Work out the finished part from the listing and answer in its coordinate system (mm). Face numbers are marked on the shaded views. A direction names the side the tool comes from. Coordinates: 2 decimals unless noted, no trailing zeros. Loops run counter-clockwise (first coordinate to the right, second up) from the corner with the lowest first, then second, coordinate; pieces in that order, holes last.
```python
from build123d import *

# Parameters (mm, degrees)
SKETCH_W        = 110
SKETCH_H        = 80
PAD_DEPTH       = 50
SKETCH001_R     = 1
POCKET_DEPTH    = 48
FILLET_R        = 2
FILLET001_R     = 2
SKETCH002_R     = 2.55
SKETCH002_W     = 11.5
SKETCH002_H     = 19.1
POCKET001_DEPTH = 5
SKETCH003_R     = 2.55
POCKET002_DEPTH = 5
BOX_W           = 15
BOX_H           = 15
BOX_DEPTH       = 15


with BuildPart() as body:
    # Sketch → Pad (new body)
    with BuildSketch(Plane.XY):
        with Locations((55, 40)):
            Rectangle(SKETCH_W, SKETCH_H)
    extrude(amount=PAD_DEPTH)

    # Sketch001 (on Face6 of Pad) → Pocket (cut)
    with BuildSketch(Plane.XY.offset(50)):
        with Locations((6, 74)):
            Circle(SKETCH001_R)
        with Locations((104, 74)):
            Circle(SKETCH001_R)
        with Locations((104, 6)):
            Circle(SKETCH001_R)
        with Locations((6, 6)):
            Circle(SKETCH001_R)
        Polygon((2, 10), (10, 10), (10, 2), (100, 2), (100, 10), (108, 10), (108, 70), (100, 70), (100, 78), (10, 78), (10, 70), (2, 70), align=None)
    extrude(amount=-POCKET_DEPTH, mode=Mode.SUBTRACT)

    # Fillet
    fillet_edges = [body.edges().sort_by_distance(p)[0] for p in [
        (0, 80, 25),
        (0, 40, 0),
        (0, 0, 25),
        (55, 0, 0),
        (110, 0, 25),
        (110, 80, 25),
        (110, 40, 0),
        (55, 80, 0),
    ]]
    fillet(fillet_edges, radius=FILLET_R)

    # Fillet001
    fillet001_edges = [body.edges().sort_by_distance(p)[0] for p in [
        (100, 10, 26),
        (100, 70, 26),
        (10, 70, 26),
        (10, 10, 26),
    ]]
    fillet(fillet001_edges, radius=FILLET001_R)

    # Sketch002 (on Face22 of Fillet001) → Pocket001 (cut)
    with BuildSketch(Plane.YZ.offset(110)):
        with Locations((15, 27.5)):
            Circle(SKETCH002_R)
        with Locations((28.75, 27.5)):
            Rectangle(SKETCH002_W, SKETCH002_H)
    extrude(amount=-POCKET001_DEPTH, mode=Mode.SUBTRACT)

    # Sketch003 (on Face18 of Pocket001) → Pocket002 (cut)
    with BuildSketch(Plane.XZ):
        with Locations((95, 27.5)):
            Circle(SKETCH003_R)
    extrude(amount=-POCKET002_DEPTH, mode=Mode.SUBTRACT)


with BuildPart() as common:
    # Box → Box (new body)
    with BuildSketch(Plane(origin=(95, 0, 35), x_dir=(1, 0, 0), z_dir=(0, 0, 1))):
        with Locations((7.5, 7.5)):
            Rectangle(BOX_W, BOX_H)
    extrude(amount=BOX_DEPTH)

    # Common: intersect Body
    add(body.part, mode=Mode.INTERSECT)


solid = common.part
```
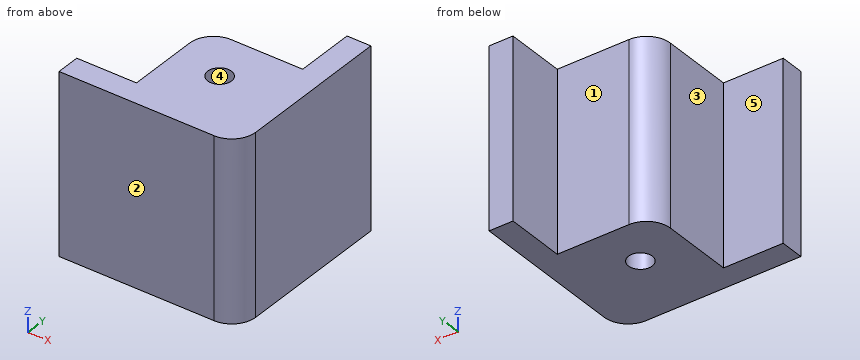
1. A cutting plane is placed at A-A, the plane y = 6. Give the vertices of the cut face in (x, z), then the cut area to 3 significant figures.
2. A cutting plane is placed at B-B, the plane x = 104. Give the vertices of the cut face in (y, z).
3. Determine the mould class of the marked faces 3, 4 and 5 for opening direction X: released by +X, released by -X, zero draft, split by the parting line, or undercut.
4. A cutting plane is placed at C-C, the plane z = 43. Give the vertices of the cut face in (x, y), then the cut area to 3 significant figures.
5. Straight lines are drawn through the part: probe 1 along Y at (x, z) = (104, 39.25); probe 2 along Y at (x, z) = (97.5, 37.25); probe 3 along X at (y, z) = (13.25, 37). For each, find the intervals that lie inside material, in ascending order.
6. A cutting plane is placed at D-D, the plane y = 12.5. Give the vertices of the cut face in (x, z), then the cut area to 3 significant figures.
7. For the marked faces 1 and 2, determine the directions among +Z, -Z, +X, -X, +Y, -Y from which every point of the face is accessible in a straight line to the end or side of a thin tool.
8. Each of these flat-tipped pins is pushed along its axis until it touches: P1, Ø3, axis at x = 105.5, z = 45, coming from the +Y side; P2, Ø3, axis at y = 4, z = 44.5, coming from the -X side; P3, Ø2.5, axis at y = 12.5, z = 42, coming from the -X side. Where does it stop, or does it pass through?
Answers below:
1. outline: (100, 35) - (103, 35) - (103, 50) - (100, 50) - close; (105, 35) - (110, 35) - (110, 50) - (105, 50) - close
1. area: 120 mm2
2. outline: (0, 35) - (5, 35) - (5, 50) - (0, 50) - close; (7, 35) - (10, 35) - (10, 50) - (7, 50) - close
3. face 3: released by -X
3. face 4: undercut
3. face 5: zero draft
4. outline: (95, 0) - (108, 0) arc R2 ccw to (110, 2) - (110, 15) - (108, 15) - (108, 10) - (102, 10) arc R2 ccw to (100, 8) - (100, 2) - (95, 2) - close; hole circle Ø2 at (104, 6)
4. area: 115 mm2
5. probe 1: y = 0 to 5, 7 to 10
5. probe 2: y = 0 to 2
5. probe 3: x = 108 to 110
6. outline: (108, 35) - (110, 35) - (110, 50) - (108, 50) - close
6. area: 30.0 mm2
7. face 1: +Z, -Z, -X, +Y
7. face 2: +Z, -Z, +X, -X, -Y
8. P1: stops at y = 10
8. P2: stops at x = 100
8. P3: stops at x = 108
